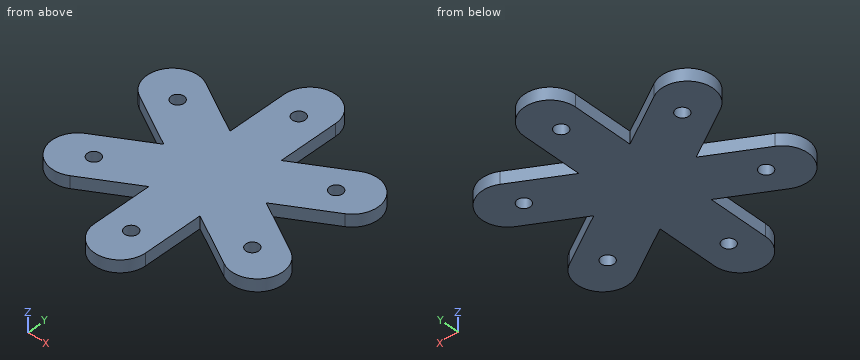
from build123d import *

# Parameters (mm, degrees)
SKETCH_1_R      = 5.25
EXTRUDE_1_DEPTH = 10


with BuildPart() as part:
    # 草图1 → 凸台-拉伸1 (new body)
    with BuildSketch(Plane.XY):
        with BuildLine():
            Line((21, 0), (21, -48.626933041))
            Line((21, -48.626933041), (63.112159322, -24.313466521))
            ThreePointArc((63.112159322, -24.313466521), (91.798692801, -32), (84.112159322, -60.686533479))
            Line((84.112159322, -60.686533479), (42, -85))
            Line((42, -85), (84.112159322, -109.313466521))
            ThreePointArc((84.112159322, -109.313466521), (91.798692801, -138), (63.112159322, -145.686533479))
            Line((63.112159322, -145.686533479), (21, -121.373066959))
            Line((21, -121.373066959), (21, -170))
            ThreePointArc((21, -170), (0, -191), (-21, -170))
            Line((-21, -170), (-21, -121.373066959))
            Line((-21, -121.373066959), (-63.112159322, -145.686533479))
            ThreePointArc((-63.112159322, -145.686533479), (-91.798692801, -138), (-84.112159322, -109.313466521))
            Line((-84.112159322, -109.313466521), (-42, -85))
            Line((-42, -85), (-84.112159322, -60.686533479))
            ThreePointArc((-84.112159322, -60.686533479), (-91.798692801, -32), (-63.112159322, -24.313466521))
            Line((-63.112159322, -24.313466521), (-21, -48.626933041))
            Line((-21, -48.626933041), (-21, 0))
            ThreePointArc((-21, 0), (0, 21), (21, 0))
        make_face()
        with Locations((0, -10)):
            Circle(SKETCH_1_R, mode=Mode.SUBTRACT)
        with Locations((64.951905284, -47.5)):
            Circle(SKETCH_1_R, mode=Mode.SUBTRACT)
        with Locations((64.951905284, -122.5)):
            Circle(SKETCH_1_R, mode=Mode.SUBTRACT)
        with Locations((0, -160)):
            Circle(SKETCH_1_R, mode=Mode.SUBTRACT)
        with Locations((-64.951905284, -122.5)):
            Circle(SKETCH_1_R, mode=Mode.SUBTRACT)
        with Locations((-64.951905284, -47.5)):
            Circle(SKETCH_1_R, mode=Mode.SUBTRACT)
    extrude(amount=EXTRUDE_1_DEPTH)


solid = part.part
Source: CAD feature listing. Evaluate the final solid. Frame: model axes, mm. Give positions to 0.01 mm unless a question says otherwise; leave off trailing zeros. Write each loop counter-clockwise with the first axis right and the second up, starting at its lowest first coordinate (ties: lowest second). Pieces come first, ordered by that corner, then holes. Notation, with made-up numbers: (7, 19.5) -> (41, 19.5) arc R7 ccw to (41, 25.5) -> close; hole circle Ø1 at (49, 3). An arc over 180 degrees is marked (long way). Return JSON: item names as keys, results as strings. Group by question number.
1. Section C-C, the plane x = -79. Output: boundary loops of the cut face in (y, z).
2. Material intervals for line 1 (Y direction, x = 0, z = 4); line 2 (Y direction, x = -64, z = 9); line 3 (X direction, y = -42, z = 4), sorted ascending. Write a range as from..to.
3. Section D-D, the plane y = -131. Output: boundary loops of the cut face in (x, z), then the cut area to 3 significant figures.
4. Section B-B, the plane z = 1.5. Output: boundary loops of the cut face in (x, y), then the cut area to 3 significant figures.
5. Pin query (flat end, axial travel): pin 1 Ø5 at (y, z) = (-151.5, 8.5) entering from -X; pin 2 Ø6.5 at (x, y) = (-64.95, -47.5) entering from -Z; pin 3 Ø1 at (y, z) = (-89, 6.5) entering from +X; pin 4 Ø2 at (x, z) = (5, 8) entering from +Y. Return the tip coordinate at first contact, or that it passes through.
6. Section A-A, the plane y = -10. Output: boundary loops of the cut face in (x, z), then the cut area to 3 significant figures.
Determined:
{
 "1": {"outline": "(-147.8, 0) -> (-106.36, 0) -> (-106.36, 10) -> (-147.8, 10) -> close; (-63.64, 0) -> (-22.2, 0) -> (-22.2, 10) -> (-63.64, 10) -> close"},
 "2": {"line 1": "y = -191..-165.25, -154.75..-15.25, -4.75..21", "line 2": "y = -146.17..-127.66, -117.34..-97.7, -72.3..-52.66, -42.34..-23.83", "line 3": "x = -94.61..-32.48, -21..21, 32.48..94.61"},
 "3": {"outline": "(-94.32, 0) -> (-37.67, 0) -> (-37.67, 10) -> (-94.32, 10) -> close; (-21, 0) -> (21, 0) -> (21, 10) -> (-21, 10) -> close; (37.67, 0) -> (94.32, 0) -> (94.32, 10) -> (37.67, 10) -> close", "area": "1,550 mm2"},
 "4": {"outline": "(-84.11, -109.31) arc R21 ccw to (-63.11, -145.69) -> (-21, -121.37) -> (-21, -170) arc R21 ccw to (21, -170) -> (21, -121.37) -> (63.11, -145.69) arc R21 ccw to (84.11, -109.31) -> (42, -85) -> (84.11, -60.69) arc R21 ccw to (63.11, -24.31) -> (21, -48.63) -> (21, 0) arc R21 ccw to (-21, 0) -> (-21, -48.63) -> (-63.11, -24.31) arc R21 ccw to (-84.11, -60.69) -> (-42, -85) -> close; hole circle Ø10.5 at (-64.95, -122.5); hole circle Ø10.5 at (-64.95, -47.5); hole circle Ø10.5 at (0, -160); hole circle Ø10.5 at (0, -10); hole circle Ø10.5 at (64.95, -122.5); hole circle Ø10.5 at (64.95, -47.5)", "area": "20,500 mm2"},
 "5": {"pin 1": "stops at x = -21", "pin 2": "passes through", "pin 3": "stops at x = 49.79", "pin 4": "stops at y = 20.62"},
 "6": {"outline": "(-21, 0) -> (-5.25, 0) -> (-5.25, 10) -> (-21, 10) -> close; (5.25, 0) -> (21, 0) -> (21, 10) -> (5.25, 10) -> close", "area": "315 mm2"}
}
